Build history of the part. All positions in model axes, mm. A direction names the side the tool comes from. Give positions to 0.01 mm unless a question says otherwise; leave off trailing zeros. Order: outer loops, then holes, each group sorted by start corner. A loop starts at its lowest first (then second) coordinate and runs counter-clockwise, first axis right, second up. Notation, with made-up numbers: M -12.75,21 L 41.25,21 A16 cw 41.25,42 Z; hole C -38,18.25 d4. An arc over 180 degrees is marked long. Use CSV: the item, a comma, the result in double quotes. Start each with the question number.
Item 1: Which spindle directions (+Z, -Z, +X, -X, +Y, -Y) get a long thin tool onto all of the face, cutting with end or side? Do faces 5 (the cylindrical face through (-13.497, 0.154, 40.472)), 6 (the flat face through (-23, 0, 32)), 7 (the flat face through (20, 0, 15)), 8 (the flat face through (-20, 0, 15)), 9 (the flat face through (20, 0, 35)). Say none if no direction does.
Item 2: Band-saw the part on D-D on z = 17. Write the cut outline in (x, y).
Item 3: Wall check: line 1 along Y through (x, z) = (-24.75, 30.5); line 2 along Y through (x, z) = (-24, 31); line 3 along Z through (x, y) = (-4, -2.25). Give the ranges that are in metal, low to high.
Item 4: Pin check, flat tips, straight feed: P1, Ø2.5, axis at x = -24.75, y = -5, coming from the +Z side; P2, Ø6, axis at x = -24, y = -2.5, coming from the -Z side; P3, Ø4, axis at x = 0, y = -3, coming from the +Z side; P4, Ø4.5, axis at y = 2.5, z = 35.5, coming from the +X side. Stop position of each tip, or through.
Item 5: Band-saw the part on C-C on y = 0. Write the cut outline in (x, z).
Item 6: Two-plate mould, pull along Y, no slides. Class faces 1 (the cylindrical face through (-5.23, 1.5, 37.99)), 2 (the cylindrical face through (26.047, 8.859, 30.986)), 3 (the cylindrical face through (-26.748, 5.088, 31.014)), 4 (the flat face through (-10, 0, 42.5)): pulls with the +Y half, pulls with the -Y half, needs draft (parallel to the pull), parting line crosses it, or undercut.
Item 7: Band-saw the part on A-A on x = 24.75. Write the cut outline in (y, z), plus the area to 3 significant figures.
Item 8: Band-saw the part on B-B on x = -10. Write the cut outline in (y, z), plus the area to 3 significant figures.
from build123d import *

# Parameters (mm, degrees)
SKETCH1_W           = 40
SKETCH1_H           = 20
BOSS_EXTRUDE2_DEPTH = 37.5
SKETCH2_W           = 2
SKETCH2_H           = 20
BOSS_EXTRUDE3_DEPTH = 7.25
SKETCH3_R           = 1.995473195
CUT_EXTRUDE1_DEPTH  = 2
FILLET3_R           = 4
SKETCH4_W           = 2
SKETCH4_H           = 20
BOSS_EXTRUDE4_DEPTH = 7.25
SKETCH5_R           = 2
CUT_EXTRUDE2_DEPTH  = 2
FILLET4_R           = 4
SKETCH6_R           = 5
BOSS_EXTRUDE5_DEPTH = 1
SKETCH7_R           = 3.5
BOSS_EXTRUDE7_DEPTH = 4


with BuildPart() as part:
    # Sketch1 → Boss-Extrude2 (new body)
    with BuildSketch(Plane.XY):
        Rectangle(SKETCH1_W, SKETCH1_H)
    extrude(amount=BOSS_EXTRUDE2_DEPTH)

    # Sketch2 → Boss-Extrude3 (add)
    with BuildSketch(Plane(origin=(20, 0, 0), x_dir=(0, 0, -1), z_dir=(1, 0, 0))):
        with Locations((-31, 0)):
            Rectangle(SKETCH2_W, SKETCH2_H)
    extrude(amount=BOSS_EXTRUDE3_DEPTH)

    # Sketch3 → Cut-Extrude1 (cut)
    with BuildSketch(Plane.XY.offset(32)):
        with Locations((24.75, -4.99913934)):
            Circle(SKETCH3_R)
        with Locations((24.75, 4.999429987)):
            Circle(SKETCH3_R)
    extrude(amount=-CUT_EXTRUDE1_DEPTH, mode=Mode.SUBTRACT)

    # Fillet3
    fillet3_edges = [part.edges().sort_by_distance(p)[0] for p in [
        (27.25, -10, 31),
        (27.25, 10, 31),
    ]]
    fillet(fillet3_edges, radius=FILLET3_R)

    # Sketch4 → Boss-Extrude4 (add)
    with BuildSketch(Plane.ZY.offset(20)):
        with Locations((31, 0)):
            Rectangle(SKETCH4_W, SKETCH4_H)
    extrude(amount=BOSS_EXTRUDE4_DEPTH)

    # Sketch5 → Cut-Extrude2 (cut)
    with BuildSketch(Plane.XY.offset(32)):
        with Locations((-24.75, 5)):
            Circle(SKETCH5_R)
        with Locations((-24.75, -5)):
            Circle(SKETCH5_R)
    extrude(amount=-CUT_EXTRUDE2_DEPTH, mode=Mode.SUBTRACT)

    # Fillet4
    fillet4_edges = [part.edges().sort_by_distance(p)[0] for p in [
        (-27.25, -10, 31),
        (-27.25, 10, 31),
    ]]
    fillet(fillet4_edges, radius=FILLET4_R)

    # Sketch6 → Boss-Extrude5 (add)
    with BuildSketch(Plane.XY.offset(37.5)):
        with Locations((-10, 0)):
            Circle(SKETCH6_R)
    extrude(amount=BOSS_EXTRUDE5_DEPTH)

    # Sketch7 → Boss-Extrude7 (add)
    with BuildSketch(Plane.XY.offset(38.5)):
        with Locations((-10, 0)):
            Circle(SKETCH7_R)
    extrude(amount=BOSS_EXTRUDE7_DEPTH)


solid = part.part
Model answer:
1,face 5,"+Z"
1,face 6,"+Z, -X, +Y, -Y"
1,face 7,"-Z, +X, +Y, -Y"
1,face 8,"-Z, -X, +Y, -Y"
1,face 9,"+Z, +X, +Y, -Y"
2,outline,"M -20,-10 L 20,-10 L 20,10 L -20,10 Z"
3,line 1,"y = -9.71 to -7, -3 to 3, 7 to 9.71"
3,line 2,"y = -9.93 to -6.85, -3.15 to 3.15, 6.85 to 9.93"
3,line 3,"z = 0 to 37.5"
4,P1,"passes through"
4,P2,"stops at z = 30"
4,P3,"stops at z = 37.5"
4,P4,"stops at x = 20"
5,outline,"M -27.25,30 L -20,30 L -20,0 L 20,0 L 20,30 L 27.25,30 L 27.25,32 L 20,32 L 20,37.5 L -5,37.5 L -5,38.5 L -6.5,38.5 L -6.5,42.5 L -13.5,42.5 L -13.5,38.5 L -15,38.5 L -15,37.5 L -20,37.5 L -20,32 L -27.25,32 Z"
6,face 1,"parting line crosses it"
6,face 2,"pulls with the +Y half"
6,face 3,"undercut"
6,face 4,"needs draft"
7,outline,"M -9.71,30 L -6.99,30 L -6.99,32 L -9.71,32 Z; M -3,30 L 3,30 L 3,32 L -3,32 Z; M 6.99,30 L 9.71,30 L 9.71,32 L 6.99,32 Z"
7,area,"22.9 mm^2"
8,outline,"M -10,0 L 10,0 L 10,37.5 L 5,37.5 L 5,38.5 L 3.5,38.5 L 3.5,42.5 L -3.5,42.5 L -3.5,38.5 L -5,38.5 L -5,37.5 L -10,37.5 Z"
8,area,"788 mm^2"
